Part print with two shaded views. Sizes in mm from the minimum x, y, z corner. A direction names the side the tool comes from. Coordinates: 2 decimals unless noted, no trailing zeros. Order: outer loops, then holes, each group sorted by start corner. A loop starts at its lowest first (then second) coordinate and runs counter-clockwise, first axis right, second up.
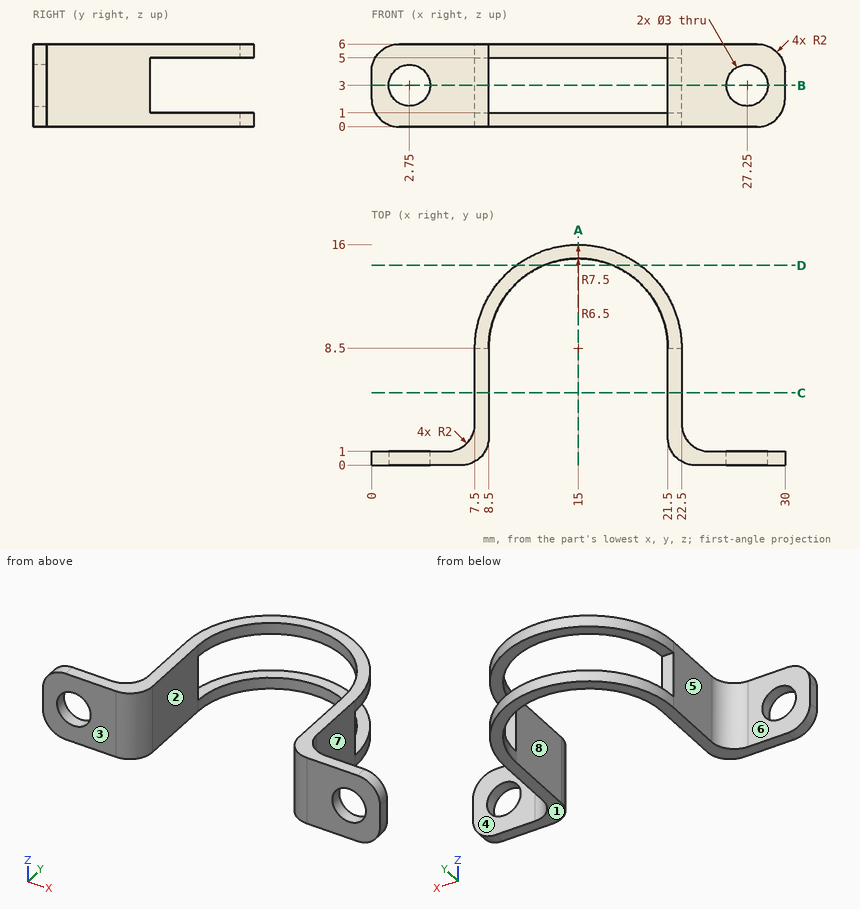
Q1. Cut at A-A on x = 15. Write the cut outline in (y, z), and give its area (3 significant figures).
Results list:
outline: (15, 0) - (16, 0) - (16, 1) - (15, 1) - close; (15, 5) - (16, 5) - (16, 6) - (15, 6) - close
area: 2.00 mm2
Q2. Mould opens along X. For the marked faces 6, 7 and 8 say: pulls with the +X half, pulls with the -X half, needs draft (parallel to the pull), parting line crosses it, or undercut.
Results list:
face 6: needs draft
face 7: pulls with the +X half
face 8: undercut
Q3. Cut at D-D on y = 14.5. Write the cut outline in (x, z).
Results list:
outline: (10.5, 0) - (12.5, 0) - (12.5, 1) - (10.5, 1) - close; (10.5, 5) - (12.5, 5) - (12.5, 6) - (10.5, 6) - close; (17.5, 0) - (19.5, 0) - (19.5, 1) - (17.5, 1) - close; (17.5, 5) - (19.5, 5) - (19.5, 6) - (17.5, 6) - close
Q4. Cut at B-B on z = 3. Write the cut outline in (x, y), and give its area (3 significant figures).
Results list:
outline: (0, 0) - (1.25, 0) - (1.25, 1) - (0, 1) - close; (4.25, 0) - (6.5, 0) arc R2 ccw to (8.5, 2) - (8.5, 8.5) - (7.5, 8.5) - (7.5, 3) arc R2 cw to (5.5, 1) - (4.25, 1) - close; (21.5, 2) arc R2 ccw to (23.5, 0) - (25.75, 0) - (25.75, 1) - (24.5, 1) arc R2 cw to (22.5, 3) - (22.5, 8.5) - (21.5, 8.5) - close; (28.75, 0) - (30, 0) - (30, 1) - (28.75, 1) - close
area: 26.0 mm2
Q5. Pin check, flat tips, straight feed: pin 1 Ø1.8 at (y, z) = (6, 3.5) entering from +X; pin 2 Ø3 at (x, z) = (21, 3) entering from +Y; pin 3 Ø3 at (x, z) = (3.5, 3.5) entering from +Y. Stop position of each tip, or through.
Results list:
pin 1: stops at x = 22.5
pin 2: stops at y = 8.5
pin 3: stops at y = 1
Q6. Cut at C-C on y = 5.25. Write the cut outline in (x, z), and give its area (3 significant figures).
Results list:
outline: (7.5, 0) - (8.5, 0) - (8.5, 6) - (7.5, 6) - close; (21.5, 0) - (22.5, 0) - (22.5, 6) - (21.5, 6) - close
area: 12.0 mm2
Q7. Which spindle directions (+Z, -Z, +X, -X, +Y, -Y) get a long thin tool onto all of the face, cutting with end or side? Do the marked faces 1, 2, 3, 4 and 5. Say none if no direction does.
Results list:
face 1: -Z, +X, -X, +Y, -Y
face 2: +Z, -Z, -Y
face 3: +Z, -Z, +X, -X, -Y
face 4: +Z, -Z, +X, +Y
face 5: +Z, -Z, -X, +Y
Q8. Wall check: line 1 along X through (y, z) = (6, 5.2); line 2 along Z through (x, y) = (2.75, 0.4); line 3 along Y through (x, z) = (25.5, 2.9). Give the ranges that are in metal, low to high.
Results list:
line 1: x = 7.5 to 8.5, 21.5 to 22.5
line 2: z = 0 to 1.5, 4.5 to 6
line 3: y = 0 to 1
